Source: three-view drawing plus pictorial views. Frame: mm from the lowest corner of the part. Coordinates: 2 decimals unless noted, no trailing zeros. Write each loop counter-clockwise with the first axis right and the second up, starting at its lowest first coordinate (ties: lowest second). Pieces come first, ordered by that corner, then holes. Notation, with made-up numbers: (75.5, 9) - (107.5, 9) arc R32 ccw to (107.5, 42) - close; hole circle Ø11 at (3.25, -37). An arc over 180 degrees is marked (long way). One line per item, written item: value.
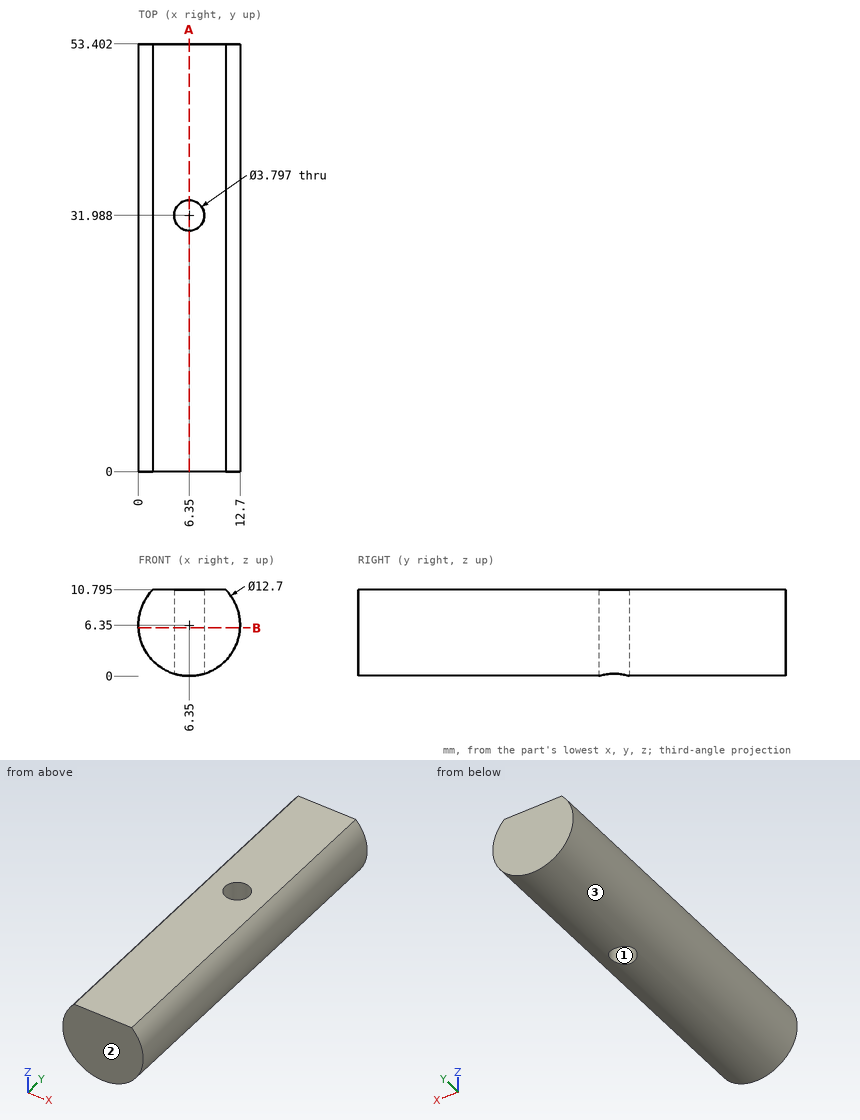
1) Material intervals for line 1 (Y direction, x = 6.35, z = 4); line 2 (Z direction, x = 6, y = 12) (1 decimal); line 3 (X direction, y = 45.5, z = 3.75), sorted ascending.
Values found:
line 1: 0 to 30.09, 33.89 to 53.4
line 2: 0 to 10.8
line 3: 0.56 to 12.14
2) Contact query for flat-ended pins moving along their axis: P1, Ø2, axis at y = 20, z = 4, coming from the +X side (1 decimal); P2, Ø1, axis at x = 10, y = 37.5, coming from the -Z side. Output: stop coordinate, or through.
Values found:
P1: x = 12.6
P2: z = 0.84
3) Section query A-A on x = 6.35. Output: boundary loops of the cut face in (y, z) (1 decimal).
Values found:
outline: (0, 0) - (30.1, 0) - (30.1, 10.8) - (0, 10.8) - close; (33.9, 0) - (53.4, 0) - (53.4, 10.8) - (33.9, 10.8) - close
4) Section query B-B on z = 6. Output: boundary loops of the cut face in (x, y).
Values found:
outline: (0.01, 0) - (12.69, 0) - (12.69, 53.4) - (0.01, 53.4) - close; hole circle Ø3.8 at (6.35, 31.99)
5) Draft query along X for the marked faces 1, 2 and 3. Return one class per face: released by +X, released by -X, zero draft, split by the parting line, or undercut.
Values found:
face 1: undercut
face 2: zero draft
face 3: split by the parting line
